Check sheet for the modelled part. Datum: model origin and axes. Units: mm. Round coordinates to 2 decimals unless told otherwise and drop trailing zeros. Loops run counter-clockwise (first coordinate to the right, second up) from the corner with the lowest first, then second, coordinate; pieces in that order, holes last. Notation, with made-up numbers: M 1,50.25 L 55,50.25 A27 ccw 55,66.25 Z; hole C 4.5,3 d9. An arc over 180 degrees is marked long. One line per question, with ' | ' between items. Start each with the question number.
(1) Thickness scan on probe 1 along X at (y, z) = (-4, 104); probe 2 along X at (y, z) = (1.5, 216); probe 3 along Y at (x, z) = (-6.5, 204.5). Record the ranges inside material, lowest first. Write a range as [from, to].
(2) Section check B-B (y = 2.5). Record the boundary of the cut face in (x, z).
(3) Section check A-A (z = 170). Record the boundary of the cut face in (x, y).
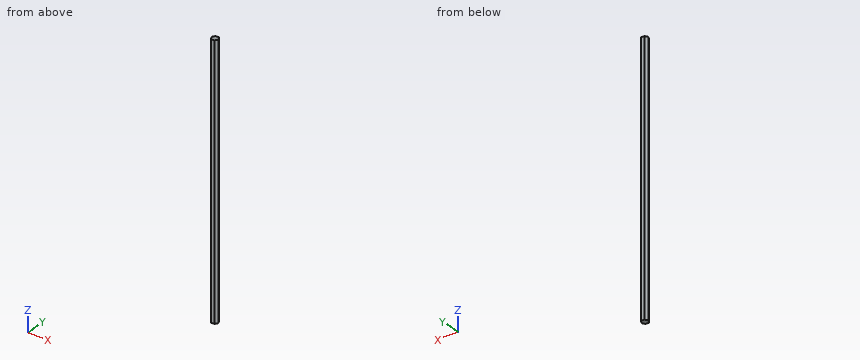
```python
from build123d import *

# Parameters (mm, degrees)
BOSS_EXTRUDE1_DEPTH      = 508
BOSS_EXTRUDE1_DEPTH_BACK = 38.1


with BuildPart() as part:
    # Sketch1 → Boss-Extrude1 (new body, two sides)
    with BuildSketch(Plane.XY) as boss_extrude1_sk:
        Polygon((7.332348419, 0), (3.666174209, 6.35), (-3.666174209, 6.35), (-7.332348419, 0), (-3.666174209, -6.35), (3.666174209, -6.35), align=None)
    extrude(amount=BOSS_EXTRUDE1_DEPTH)
    extrude(boss_extrude1_sk.sketch, amount=-BOSS_EXTRUDE1_DEPTH_BACK)


solid = part.part
```
The answers:
1) probe 1: [-5.02, 5.02] | probe 2: [-6.47, 6.47] | probe 3: [-1.44, 1.44]
2) outline: M -5.89,-38.1 L 5.89,-38.1 L 5.89,508 L -5.89,508 Z
3) outline: M -7.33,0 L -3.67,-6.35 L 3.67,-6.35 L 7.33,0 L 3.67,6.35 L -3.67,6.35 Z
